Verification items for the finished model (mm, model axes). Coordinates: 2 decimals unless noted, no trailing zeros. Loops run counter-clockwise (first coordinate to the right, second up) from the corner with the lowest first, then second, coordinate; pieces in that order, holes last. Notation, with made-up numbers: (67.5, 85) - (121.5, 85) arc R28 ccw to (121.5, 119) - close; hole circle Ø6 at (76, 50.25). An arc over 180 degrees is marked (long way). Answer as CSV lines item,"result". Start each with the question number.
1. Cross-section at A-A (y = 34.5). Enter the section's corners in (x, z).
2. Gauge pin test, flat end, axial feed: P1, Ø8, axis at x = -22, y = -18.5, coming from the -Z side. Record the tip position at first contact, or that the pin passes through.
3. Material ranges on line 1 (Y direction, x = 34.5, z = 0.4); line 2 (X direction, y = 34, z = 0.9), recorded low to high. Write a range as [from, to].
```python
from build123d import *

# Parameters (mm, degrees)
SKETCH_1_W      = 74
SKETCH_1_H      = 74
SKETCH_1_R      = 1.1
EXTRUDE_1_DEPTH = 1
FILLET_1_R      = 1.5


with BuildPart() as part:
    # 草图1 → 凸台-拉伸1 (new body)
    with BuildSketch(Plane.XY):
        Rectangle(SKETCH_1_W, SKETCH_1_H)
        with Locations((-34.5, 34.5)):
            Circle(SKETCH_1_R, mode=Mode.SUBTRACT)
        with Locations((34.5, 34.5)):
            Circle(SKETCH_1_R, mode=Mode.SUBTRACT)
        with Locations((34.5, -34.5)):
            Circle(SKETCH_1_R, mode=Mode.SUBTRACT)
        with Locations((-34.5, -34.5)):
            Circle(SKETCH_1_R, mode=Mode.SUBTRACT)
    extrude(amount=EXTRUDE_1_DEPTH)

    # 圆角1
    fillet_1_edges = [part.edges().sort_by_distance(p)[0] for p in [
        (37, -37, 0.5),
        (-37, -37, 0.5),
        (-37, 37, 0.5),
        (37, 37, 0.5),
    ]]
    fillet(fillet_1_edges, radius=FILLET_1_R)


solid = part.part
```
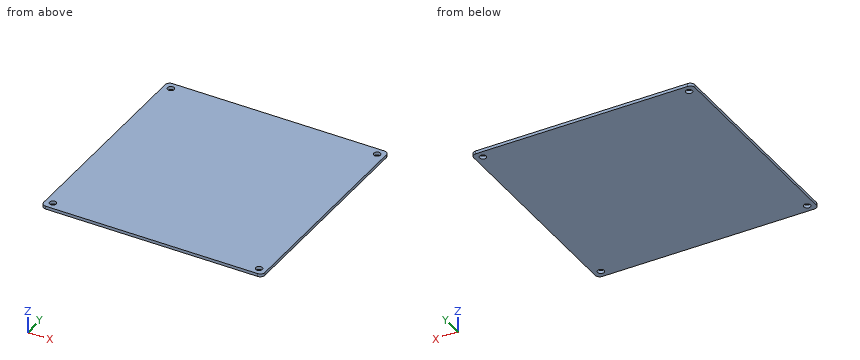
Values follow:
1,outline,"(-37, 0) - (-35.6, 0) - (-35.6, 1) - (-37, 1) - close; (-33.4, 0) - (33.4, 0) - (33.4, 1) - (-33.4, 1) - close; (35.6, 0) - (37, 0) - (37, 1) - (35.6, 1) - close"
2,P1,"stops at z = 0"
3,line 1,"y = [-37, -35.6], [-33.4, 33.4], [35.6, 37]"
3,line 2,"x = [-37, -35.48], [-33.52, 33.52], [35.48, 37]"
